CAD build for the part. Positions are in the model's coordinates, mm. Face numbers are marked on the shaded views. A direction names the side the tool comes from. Coordinates: 2 decimals unless noted, no trailing zeros. Write each loop counter-clockwise with the first axis right and the second up, starting at its lowest first coordinate (ties: lowest second). Pieces come first, ordered by that corner, then holes.
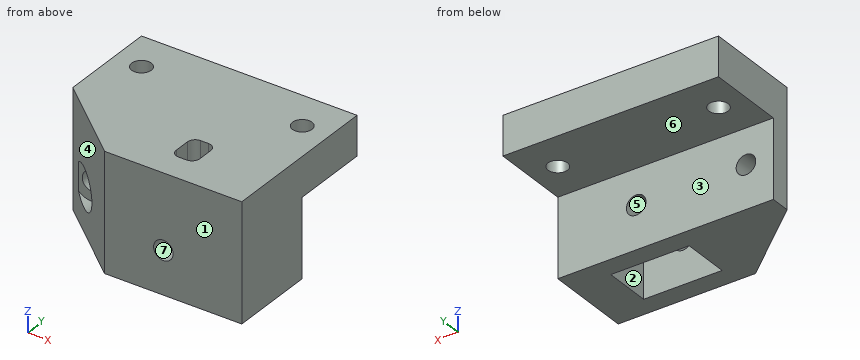
Autodesk Inventor part; units mm, degrees
ref_plane "YZ Plane" through (0, 0, 0) normal (1, 0, 0) x (0, 1, 0)
ref_plane "XZ Plane" through (0, 0, 0) normal (0, 1, 0) x (-1, 0, 0)
ref_plane "XY Plane" through (0, 0, 0) normal (0, 0, 1) x (1, 0, 0)
sketch "Boceto1" plane through (0, 0, 0) normal (0, 0, 1) x (1, 0, 0)
  line L0 (-27.5, 10) -> (27.5, 10)
  line L1 (27.5, 10) -> (27.5, -10)
  line L2 (27.5, -10) -> (-27.5, -10)
  line L3 (-27.5, -10) -> (-27.5, 10)
  line L4 (0, 0) -> (0, 1.7227)
  line L5 (0, 0) -> (-2.1619, 0)
  line L6 (27.5, -10) -> (-2.5, -10)
  line L7 (-2.5, -10) -> (-2.5, -27)
  line L8 (-2.5, -27) -> (27.5, -27)
  line L9 (27.5, -27) -> (27.5, -10)
  circle A0 centre (20.5, 0) radius 2.5
  circle A1 centre (-20.5, 0) radius 2.5
  point P0 (-2.5, -10)
  dimension "d14" = 55
  dimension "d15" = 20
  dimension "d16" = 30
  dimension "d17" = 17
  dimension "d18" = 5
  dimension "d19" = 5
  dimension "d20" = 7
  dimension "d21" = 7
extrude "Extrusión1" add sketch "Boceto1" along normal blind 10
sketch "Boceto2" plane through (-2.5, -27, 0) normal (0, -1, 0) x (1, 0, 0)
  line L0 (30, 10) -> (-25, 10)
  line L1 (30, 10) -> (0, 10)
  line L2 (0, 10) -> (0, -20)
  line L3 (0, -20) -> (30, -20)
  line L4 (30, -20) -> (30, 10)
  line L5 (0, 0) -> (0, 10)
  point P0 (2.5, 0)
  point P1 (0, 10)
  dimension "d22" = 30
extrude "Extrusión2" add sketch "Boceto2" along normal blind 5
sketch "Boceto4" plane through (-27.5, -10, 0) normal (-1, 0, 0) x (0, 0, 1)
  line L0 (0, 0) -> (0, -17)
  line L1 (10, 20) -> (10, 0)
  line L2 (10, 0) -> (-20, 0)
  line L3 (-20, 0) -> (-20, -5)
  line L4 (-20, -5) -> (10, -5)
  line L5 (10, -5) -> (10, 0)
  line L6 (10, -22) -> (-20, -22)
  point P0 (0, 10)
  dimension "d32" = 5
  dimension "d43" = 30
  dimension "d44" = 30
extrude "Extrusión4" add sketch "Boceto4" against normal up to surface (55 mm away)
sketch "Boceto5" plane through (-2.5, -32, 0) normal (0, -1, 0) x (1, 0, 0)
  circle A0 centre (10, -9) radius 2.5
  line L0 (30, -20) -> (30, 10)
  line L1 (0, -20) -> (30, -20)
  line L2 (-25, -20) -> (30, -20)
  line L3 (-25, -20) -> (-25, 10)
  line L4 (-25, 0) -> (30, 0)
  point P0 (2.5, 0)
  point P1 (0, 0)
  dimension "d33" = 5
  dimension "d34" = 20
  dimension "d41" = 9
extrude "Extrusión5" cut sketch "Boceto5" against normal up to surface (22 mm away) contours A0
sketch "Boceto8" plane through (-27.5, -15, -20) normal (0, -1, 0) x (1, 0, 0)
  line L0 (0, 30) -> (25, 30)
  line L1 (0, 0) -> (55, 0)
  line L2 (25, 30) -> (20, 30)
  line L3 (20, 30) -> (20, 0)
  line L4 (20, 0) -> (25, 0)
  line L5 (25, 0) -> (25, 30)
  line L6 (25, 20) -> (55, 20)
  line L7 (45, 20) -> (55, 20)
  line L8 (55, 20) -> (55, 0)
  line L9 (55, 0) -> (45, 0)
  line L10 (45, 0) -> (45, 20)
  line L11 (55, 0) -> (55, 20)
  point P0 (27.5, 20)
  point P1 (45, 0)
  point P2 (25, 0)
  point P3 (20, 30)
  dimension "d54" = 5
  dimension "d56" = 0
  dimension "d69" = 10
extrude "Extrusión8" add sketch "Boceto8" along normal up to surface (17 mm away) contours L0 L5 L1 L3 | L6 L8 L1 L10
sketch "Boceto9" plane through (0, 0, 10) normal (0, 0, 1) x (1, 0, 0)
  line L0 (27.5, -32) -> (-7.5, -32)
  line L1 (-27.5, 10) -> (-27.5, -15)
  line L2 (-7.5, -32) -> (-27.5, -15)
  line L3 (-27.5, -15) -> (-7.5, -15)
  line L4 (-7.5, -15) -> (-7.5, -32)
  point P0 (0, 0)
extrude "Extrusión9" add sketch "Boceto9" against normal up to surface (30 mm away)
sketch "Boceto10" plane through (-2.5, -32, 0) normal (0, -1, 0) x (1, 0, 0)
  circle A0 centre (-18, -9) radius 2.5
  line L0 (-25, 10) -> (-5, 10)
  line L1 (-25, -20) -> (-25, 10)
  point P0 (2.5, 0)
  dimension "d61" = 5
  dimension "d62" = 19
  dimension "d63" = 7
extrude "Extrusión10" cut sketch "Boceto10" against normal up to surface (22 mm away)
sketch "Boceto11" plane through (-2.5, -32, 0) normal (0, -1, 0) x (1, 0, 0)
  circle A0 centre (-18, -9) radius 2.5
  circle A1 centre (-18, -9) radius 5
  point P0 (2.5, 0)
  dimension "d66" = 10
extrude "Extrusión11" cut sketch "Boceto11" against normal blind 14 contours A0 | A1
sketch "Boceto12" plane through (0, 0, 10) normal (0, 0, 1) x (1, 0, 0)
  line L0 (7.5, -25) -> (4.5, -25)
  line L1 (4.5, -25) -> (4.5, -17)
  line L2 (4.5, -17) -> (7.5, -17)
  line L3 (7.5, -17) -> (7.5, -25)
  line L4 (7.5, -17) -> (10.5, -17)
  line L5 (10.5, -17) -> (10.5, -25)
  line L6 (7.5, -25) -> (7.5, -17)
  line L7 (27.5, -32) -> (-7.5, -32)
  line L8 (7.5, -25) -> (10.5, -25)
  line L9 (-27.5, -10) -> (27.5, -10)
  point P0 (0, 0)
  dimension "d70" = 3
  dimension "d72" = 3
  dimension "d77" = 7
  dimension "d78" = 8
extrude "Extrusión12" cut sketch "Boceto12" against normal up to surface (10 mm away)
fillet "Empalme4" radius 2 4 edges at (10.5, -17, 5) (4.5, -17, 5) (10.5, -25, 5) (4.5, -25, 5)
equation "\"d19\" = d18"
equation "\"d20\" = d21"
equation "\"d44\" = d43"
equation "\"d72\" = d70"
properties part number "Soporte Idler Z" material "Hormigón reforzado con fibra de vidrio"
Item 1: Two-plate mould, pull along X, no slides. Class the marked faces 4, 5, 6 and 7: +X half, -X half, draft (parallel to the pull), parting line (faces both ways), or undercut.
Item 2: Saw through at A-A, the plane z = -9. Write the cut outline in (x, y), and give its area (3 significant figures).
Item 3: Saw through at D-D, the plane z = -0.75. Write the cut outline in (x, y), and give its area (3 significant figures).
Item 4: Flat gauge pins, fed straight in: pin 1 Ø1.2 at (y, z) = (-20.5, 3) entering from -X; pin 2 Ø12 at (x, y) = (-10.5, -1.5) entering from -Z; pin 3 Ø10 at (x, z) = (11.5, -10) entering from +Y. Where does each tip first touch, or does it go through?
Item 5: Saw through at C-C, the plane y = 0. Write the cut outline in (x, z).
Item 6: Which spindle directions (+Z, -Z, +X, -X, +Y, -Y) get a long thin tool onto all of the face, cutting with end or side? Do the marked faces 1, 2 and 3. Say none if no direction does.
Item 7: Saw through at B-B, the plane x = 20.5. Write the cut outline in (y, z).
Item 8: Wall check: line 1 along Y through (x, z) = (-0.5, -16.25); line 2 along X through (y, z) = (-19.5, -9); line 3 along Z through (x, y) = (0, -21.5). Give the ranges that are in metal, low to high.
Working result:
1. face 4: -X half
1. face 5: undercut
1. face 6: draft
1. face 7: undercut
2. outline: (-27.5, -15) - (-23.97, -18) - (-23, -18) - (-23, -10) - (-27.5, -10) - close; (-18, -18) - (-15.5, -18) - (-15.5, -25.2) - (-7.5, -32) - (5, -32) - (5, -27) - (-2.5, -27) - (-2.5, -15) - (5, -15) - (5, -10) - (-18, -10) - close; (10, -32) - (27.5, -32) - (27.5, -10) - (10, -10) - (10, -15) - (17.5, -15) - (17.5, -27) - (10, -27) - close
2. area: 680 mm2
3. outline: (-27.5, -15) - (-7.5, -32) - (27.5, -32) - (27.5, -10) - (-27.5, -10) - close; hole (-2.5, -27) - (17.5, -27) - (17.5, -15) - (-2.5, -15) - close
3. area: 800 mm2
4. pin 1: stops at x = -21.74
4. pin 2: stops at z = 0
4. pin 3: stops at y = -10
5. outline: (-27.5, 0) - (-23, 0) - (-23, 10) - (-27.5, 10) - close; (-18, 0) - (18, 0) - (18, 10) - (-18, 10) - close; (23, 0) - (27.5, 0) - (27.5, 10) - (23, 10) - close
6. face 1: +Z, -Z, +X, -X, -Y
6. face 2: -Z
6. face 3: -Z, +X, -X, +Y
7. outline: (-32, -20) - (-10, -20) - (-10, 0) - (-2.5, 0) - (-2.5, 10) - (-32, 10) - close; (2.5, 0) - (10, 0) - (10, 10) - (2.5, 10) - close
8. line 1: y = -32 to -27, -15 to -10
8. line 2: x = -15.5 to -2.5, 17.5 to 27.5
8. line 3: z = 0 to 10
